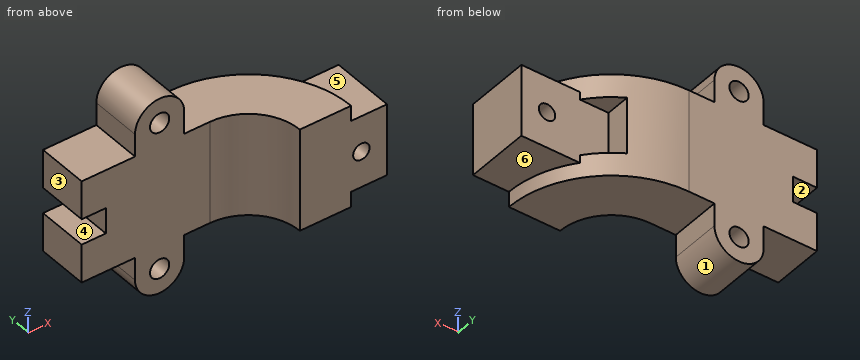
from build123d import *

# Parameters (mm, degrees)
BOSS_EXTRUDE1_DEPTH = 6.35
BOSS_EXTRUDE2_START = 6.35
SKETCH1_3_W         = 11.938
SKETCH1_3_H         = 19.05
SKETCH1_3_H_2       = 6.35
BOSS_EXTRUDE2_DEPTH = 7.62
BOSS_EXTRUDE3_START = 13.97
SKETCH1_7_W         = 11.938
SKETCH1_7_H         = 19.05
SKETCH1_7_H_2       = 6.35
BOSS_EXTRUDE3_DEPTH = 3.81
BOSS_EXTRUDE4_START = 17.78
SKETCH1_10_W        = 11.938
SKETCH1_10_H        = 6.35
SKETCH1_10_H_2      = 19.05
BOSS_EXTRUDE4_DEPTH = 7.62
SKETCH2_R           = 4.7625
BOSS_EXTRUDE5_DEPTH = 25.4
SKETCH3_R           = 4.064
CUT_EXTRUDE1_DEPTH  = 32.75


with BuildPart() as part:
    # Sketch1 → Boss-Extrude1 (new body)
    with BuildSketch(Plane.XY):
        with BuildLine():
            ThreePointArc((0, 25.4), (17.960512242, 17.960512242), (25.4, 0))
            Line((25.4, 0), (25.4, 31.75))
            Line((25.4, 31.75), (-51.562, 31.75))
            Line((-51.562, 31.75), (-51.562, 25.4))
            Line((-51.562, 25.4), (0, 25.4))
        make_face()
        with BuildLine():
            Line((-51.562, 31.75), (25.4, 31.75))
            Line((25.4, 31.75), (25.4, 43.994090512))
            ThreePointArc((25.4, 43.994090512), (13.148007491, 49.069031975), (0, 50.8))
            Line((0, 50.8), (-51.562, 50.8))
            Line((-51.562, 50.8), (-51.562, 31.75))
        make_face()
        with BuildLine():
            Line((25.4, 31.75), (25.4, 0))
            Line((25.4, 0), (50.8, 0))
            ThreePointArc((50.8, 0), (47.933033778, 16.824514045), (39.65573729, 31.75))
            Line((39.65573729, 31.75), (25.4, 31.75))
        make_face()
        with BuildLine():
            ThreePointArc((39.65573729, 31.75), (47.933033778, 16.824514045), (50.8, 0))
            Line((50.8, 0), (68.58, 0))
            Line((68.58, 0), (68.58, 31.75))
            Line((68.58, 31.75), (39.65573729, 31.75))
        make_face()
    boss_extrude1 = extrude(amount=BOSS_EXTRUDE1_DEPTH)

    # Sketch1<3> → Boss-Extrude2 (add)
    with BuildSketch(Plane.XY.offset(BOSS_EXTRUDE2_START)):
        with BuildLine():
            Line((-51.562, 31.75), (25.4, 31.75))
            Line((25.4, 31.75), (25.4, 43.994090512))
            ThreePointArc((25.4, 43.994090512), (13.148007491, 49.069031975), (0, 50.8))
            Line((0, 50.8), (-51.562, 50.8))
            Line((-51.562, 50.8), (-51.562, 31.75))
        make_face()
        with BuildLine():
            ThreePointArc((0, 25.4), (17.960512242, 17.960512242), (25.4, 0))
            Line((25.4, 0), (25.4, 31.75))
            Line((25.4, 31.75), (-51.562, 31.75))
            Line((-51.562, 31.75), (-51.562, 25.4))
            Line((-51.562, 25.4), (0, 25.4))
        make_face()
        with Locations((-57.531, 41.275)):
            Rectangle(SKETCH1_3_W, SKETCH1_3_H)
        with BuildLine():
            Line((25.4, 31.75), (25.4, 0))
            Line((25.4, 0), (50.8, 0))
            ThreePointArc((50.8, 0), (47.933033778, 16.824514045), (39.65573729, 31.75))
            Line((39.65573729, 31.75), (25.4, 31.75))
        make_face()
        with BuildLine():
            ThreePointArc((39.65573729, 31.75), (47.933033778, 16.824514045), (50.8, 0))
            Line((50.8, 0), (68.58, 0))
            Line((68.58, 0), (68.58, 31.75))
            Line((68.58, 31.75), (39.65573729, 31.75))
        make_face()
        with Locations((-57.531, 28.575)):
            Rectangle(SKETCH1_3_W, SKETCH1_3_H_2)
    boss_extrude2 = extrude(amount=BOSS_EXTRUDE2_DEPTH)

    # Sketch1<7> → Boss-Extrude3 (add)
    with BuildSketch(Plane.XY.offset(BOSS_EXTRUDE3_START)):
        with BuildLine():
            Line((-51.562, 31.75), (25.4, 31.75))
            Line((25.4, 31.75), (25.4, 43.994090512))
            ThreePointArc((25.4, 43.994090512), (13.148007491, 49.069031975), (0, 50.8))
            Line((0, 50.8), (-51.562, 50.8))
            Line((-51.562, 50.8), (-51.562, 31.75))
        make_face()
        with BuildLine():
            ThreePointArc((0, 25.4), (17.960512242, 17.960512242), (25.4, 0))
            Line((25.4, 0), (25.4, 31.75))
            Line((25.4, 31.75), (-51.562, 31.75))
            Line((-51.562, 31.75), (-51.562, 25.4))
            Line((-51.562, 25.4), (0, 25.4))
        make_face()
        with BuildLine():
            Line((25.4, 31.75), (25.4, 0))
            Line((25.4, 0), (50.8, 0))
            ThreePointArc((50.8, 0), (47.933033778, 16.824514045), (39.65573729, 31.75))
            Line((39.65573729, 31.75), (25.4, 31.75))
        make_face()
        with BuildLine():
            Line((25.4, 43.994090512), (25.4, 31.75))
            Line((25.4, 31.75), (39.65573729, 31.75))
            ThreePointArc((39.65573729, 31.75), (33.09896791, 38.536973458), (25.4, 43.994090512))
        make_face()
        with Locations((-57.531, 41.275)):
            Rectangle(SKETCH1_7_W, SKETCH1_7_H)
        with Locations((-57.531, 28.575)):
            Rectangle(SKETCH1_7_W, SKETCH1_7_H_2)
        with BuildLine():
            ThreePointArc((39.65573729, 31.75), (47.933033778, 16.824514045), (50.8, 0))
            Line((50.8, 0), (68.58, 0))
            Line((68.58, 0), (68.58, 31.75))
            Line((68.58, 31.75), (39.65573729, 31.75))
        make_face()
    boss_extrude3 = extrude(amount=BOSS_EXTRUDE3_DEPTH)

    # Sketch1<10> → Boss-Extrude4 (add)
    with BuildSketch(Plane.XY.offset(BOSS_EXTRUDE4_START)):
        with BuildLine():
            Line((-51.562, 31.75), (25.4, 31.75))
            Line((25.4, 31.75), (25.4, 43.994090512))
            ThreePointArc((25.4, 43.994090512), (13.148007491, 49.069031975), (0, 50.8))
            Line((0, 50.8), (-51.562, 50.8))
            Line((-51.562, 50.8), (-51.562, 31.75))
        make_face()
        with BuildLine():
            ThreePointArc((0, 25.4), (17.960512242, 17.960512242), (25.4, 0))
            Line((25.4, 0), (25.4, 31.75))
            Line((25.4, 31.75), (-51.562, 31.75))
            Line((-51.562, 31.75), (-51.562, 25.4))
            Line((-51.562, 25.4), (0, 25.4))
        make_face()
        with Locations((-57.531, 28.575)):
            Rectangle(SKETCH1_10_W, SKETCH1_10_H)
        with Locations((-57.531, 41.275)):
            Rectangle(SKETCH1_10_W, SKETCH1_10_H_2)
        with BuildLine():
            Line((25.4, 43.994090512), (25.4, 31.75))
            Line((25.4, 31.75), (39.65573729, 31.75))
            ThreePointArc((39.65573729, 31.75), (33.09896791, 38.536973458), (25.4, 43.994090512))
        make_face()
        with BuildLine():
            Line((25.4, 31.75), (25.4, 0))
            Line((25.4, 0), (50.8, 0))
            ThreePointArc((50.8, 0), (47.933033778, 16.824514045), (39.65573729, 31.75))
            Line((39.65573729, 31.75), (25.4, 31.75))
        make_face()
    boss_extrude4 = extrude(amount=BOSS_EXTRUDE4_DEPTH)

    # Mirror7: Boss-Extrude1, Boss-Extrude2, Boss-Extrude3, Boss-Extrude4 across plane
    add(boss_extrude1.mirror(Plane.XY))
    add(boss_extrude2.mirror(Plane.XY))
    add(boss_extrude3.mirror(Plane.XY))
    add(boss_extrude4.mirror(Plane.XY))

    # Sketch2 → Boss-Extrude5 (add)
    with BuildSketch(Plane(origin=(0, 50.8, 0), x_dir=(1, 0, 0), z_dir=(0, 1, 0))):
        with BuildLine():
            Line((-12.7, 25.4), (-12.7, 36.576))
            ThreePointArc((-12.7, 36.576), (-24.892, 48.768), (-37.084, 36.576))
            Line((-37.084, 36.576), (-37.084, 25.4))
            Line((-37.084, 25.4), (-12.7, 25.4))
        make_face()
        with Locations((-24.892, 36.576)):
            Circle(SKETCH2_R, mode=Mode.SUBTRACT)
        with BuildLine():
            Line((-37.084, -25.4), (-37.084, -36.576))
            ThreePointArc((-37.084, -36.576), (-24.892, -48.768), (-12.7, -36.576))
            Line((-12.7, -36.576), (-12.7, -25.4))
            Line((-12.7, -25.4), (-37.084, -25.4))
        make_face()
        with Locations((-24.892, -36.576)):
            Circle(SKETCH2_R, mode=Mode.SUBTRACT)
    extrude(amount=-BOSS_EXTRUDE5_DEPTH)

    # Sketch3 → Cut-Extrude1 (cut, through all)
    with BuildSketch(Plane(origin=(0, 31.75, 0), x_dir=(1, 0, 0), z_dir=(0, 1, 0))):
        with Locations((55.88, 0)):
            Circle(SKETCH3_R)
    extrude(amount=-CUT_EXTRUDE1_DEPTH, mode=Mode.SUBTRACT)


solid = part.part
The listing builds one solid part. Answer for the finished solid, in the listing's coordinates (mm). Face numbers are marked on the shaded views. A direction names the side the tool comes from. Round coordinates to 2 decimals unless told otherwise and drop trailing zeros. Loops run counter-clockwise (first coordinate to the right, second up) from the corner with the lowest first, then second, coordinate; pieces in that order, holes last. Notation, with made-up numbers: M -7,80.5 L 19,80.5 A36 cw 19,114.5 Z; hole C 61.5,-22.5 d1. An arc over 180 degrees is marked long. Write each question's results on one line, items separated by ' | '. Start each with the question number.
1) Find section C-C on y = 22.5. Write down the section's boundary in (x, z), plus the area to 3 significant figures.
2) Find section B-B on z = 0. Write down the section's boundary in (x, y), plus the area to 3 significant figures.
3) Find section D-D on x = -25. Write down the section's boundary in (y, z).
4) Find section A-A on x = 55.88. Write down the section's boundary in (y, z), plus the area to 3 significant figures.
5) Straight lines are drawn through the part: probe 1 along Z at (x, y) = (55.88, 20); probe 2 along Z at (x, y) = (22, 33.5); probe 3 along X at (y, z) = (35, -29.5). For each, find the intervals that lie inside material, in ascending order.
6) Each of these flat-tipped pins is pushed along its axis until it touches: pin 1 (10 mm diameter, centred on x = 35, y = 39.5, fed in from +Z); pin 2 (20.5 mm diameter, centred on x = -51, y = 35, fed in from -Z); pin 3 (6 mm diameter, centred on y = 21.5, z = 33, fed in from +X); pin 4 (5.5 mm diameter, centred on y = 39, z = -29.5, fed in from -X). Where does it stop, or does it pass through?
7) Determine the mould class of the marked faces 1, 2 and 3 for opening direction Z: pulls with the +Z half, pulls with the -Z half, needs draft (parallel to the pull), parting line crosses it, or undercut.
8) Which of the six approach directions +Z, -Z, +X, -X, +Y, -Y give full straight-line access (tool end or side, diameter ignored) to the marked faces 4, 5 and 6?
Final values:
1) outline: M 11.79,-25.4 L 45.55,-25.4 L 45.55,-17.78 L 68.58,-17.78 L 68.58,17.78 L 45.55,17.78 L 45.55,25.4 L 11.79,25.4 Z; hole C 55.88,0 d8.13 | area: 2,480 mm²
2) outline: M -51.56,25.4 L 0,25.4 A25.4 cw 25.4,0 L 51.82,0 L 51.82,31.75 L 25.4,31.75 L 25.4,43.99 A50.8 ccw 0,50.8 L -51.56,50.8 Z; M 59.94,0 L 68.58,0 L 68.58,31.75 L 59.94,31.75 Z | area: 3,150 mm²
3) outline: M 25.4,-48.77 L 50.8,-48.77 L 50.8,-41.34 L 25.4,-41.34 Z; M 25.4,-31.81 L 50.8,-31.81 L 50.8,31.81 L 25.4,31.81 Z; M 25.4,41.34 L 50.8,41.34 L 50.8,48.77 L 25.4,48.77 Z
4) outline: M 0,-17.78 L 31.75,-17.78 L 31.75,-4.06 L 0,-4.06 Z; M 0,4.06 L 31.75,4.06 L 31.75,17.78 L 0,17.78 Z | area: 871 mm²
5) probe 1: -17.78 to -4.06, 4.06 to 17.78 | probe 2: -25.4 to 25.4 | probe 3: -37.08 to -12.7
6) pin 1: z = 25.4 | pin 2: z = -25.4 | pin 3: through | pin 4: x = -37.08
7) face 1: pulls with the -Z half | face 2: undercut | face 3: needs draft
8) face 4: -X, +Y, -Y | face 5: +Z, +X, +Y | face 6: -Z, +X, +Y
